from build123d import *

# Parameters (mm, degrees)
ESQUISSE1_W                     = 98
ESQUISSE1_H                     = 110
ESQUISSE1_W_2                   = 78
ESQUISSE1_H_2                   = 90
BOSS_EXTRU_1_DEPTH              = 5
ESQUISSE2_R                     = 5
ESQUISSE2_R_2                   = 2.5
BOSS_EXTRU_2_DEPTH              = 10
ESQUISSE3_R                     = 2.5
ENL_V_MAT_EXTRU_1_DEPTH         = 10
R_P_TITION_LIN_AIRE3_COUNT      = 2
R_P_TITION_LIN_AIRE3_PITCH      = 88
R_P_TITION_LIN_AIRE3_COUNT_DIR2 = 2
R_P_TITION_LIN_AIRE3_PITCH_DIR2 = 90
CONG_1_R                        = 5


with BuildPart() as part:
    # Esquisse1 → Boss.-Extru.1 (new body)
    with BuildSketch(Plane.XY):
        with Locations((54.666666667, 49.166666667)):
            Rectangle(ESQUISSE1_W, ESQUISSE1_H)
        with Locations((54.666666667, 49.166666667)):
            Rectangle(ESQUISSE1_W_2, ESQUISSE1_H_2, mode=Mode.SUBTRACT)
    extrude(amount=BOSS_EXTRU_1_DEPTH)

    # Esquisse2 → Boss.-Extru.2 (add)
    with BuildSketch(Plane(origin=(103.666666667, 0, 0), x_dir=(0, 0, -1), z_dir=(1, 0, 0))):
        with Locations((-7.1, 94.166666667)):
            Circle(ESQUISSE2_R)
        with Locations((-7.1, 94.166666667)):
            Circle(ESQUISSE2_R_2, mode=Mode.SUBTRACT)
    boss_extru_2 = extrude(amount=-BOSS_EXTRU_2_DEPTH)

    # Esquisse3 → Enlèv. mat.-Extru.1 (cut)
    with BuildSketch(Plane(origin=(103.666666667, 0, 0), x_dir=(0, 0, -1), z_dir=(1, 0, 0))):
        with Locations((-7.1, 94.166666667)):
            Circle(ESQUISSE3_R)
    enl_v_mat_extru_1 = extrude(amount=-ENL_V_MAT_EXTRU_1_DEPTH, mode=Mode.SUBTRACT)

    # Répétition linéaire3: Boss.-Extru.2, Enl_v. mat.-Extru.1 2 × 2
    with Locations(*[(-i * R_P_TITION_LIN_AIRE3_PITCH, -j * R_P_TITION_LIN_AIRE3_PITCH_DIR2, 0) for i in range(R_P_TITION_LIN_AIRE3_COUNT) for j in range(R_P_TITION_LIN_AIRE3_COUNT_DIR2) if (i, j) != (0, 0)]):
        add(boss_extru_2)
        add(enl_v_mat_extru_1, mode=Mode.SUBTRACT)

    # Congé1
    cong_1_edges = [part.edges().sort_by_distance(p)[0] for p in [
        (10.666666667, -0.370953855, 5),
        (10.666666667, 8.704287188, 5),
        (98.666666667, 89.629046145, 5),
        (98.666666667, 98.704287188, 5),
        (98.666666667, -0.370953855, 5),
        (98.666666667, 8.704287188, 5),
        (10.666666667, 89.629046145, 5),
        (10.666666667, 98.704287188, 5),
    ]]
    fillet(cong_1_edges, radius=CONG_1_R)


solid = part.part
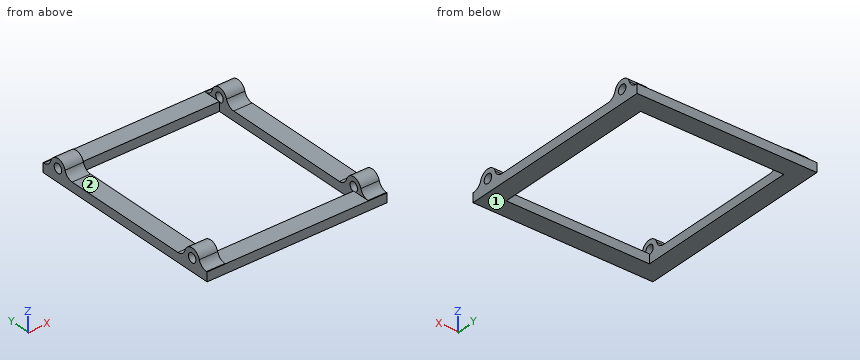
Part model, mm, in its own coordinate system. Face numbers are marked on the shaded views. Round coordinates to 2 decimals unless told otherwise and drop trailing zeros. Loops run counter-clockwise (first coordinate to the right, second up) from the corner with the lowest first, then second, coordinate; pieces in that order, holes last. Notation, with made-up numbers: (41.5, 89.5) - (85.5, 89.5) arc R23 ccw to (85.5, 113.5) - close; hole circle Ø3 at (-36.5, 59). An arc over 180 degrees is marked (long way). Answer as a JSON object with one key per item and string values.
Item 1: Band-saw the part on A-A on x = 57.5. List the corners of the cut face in (y, z).
Output:
{"outline": "(-5.83, 0) - (4.17, 0) - (4.17, 5) - (-5.83, 5) - close; (94.17, 0) - (104.17, 0) - (104.17, 5) - (94.17, 5) - close"}
Item 2: Band-saw the part on B-B on y = 49. List the corners of the cut face in (x, z), plus the area to 3 significant figures.
Output:
{"outline": "(5.67, 0) - (15.67, 0) - (15.67, 5) - (5.67, 5) - close; (93.67, 0) - (103.67, 0) - (103.67, 5) - (93.67, 5) - close", "area": "100 mm2"}
Item 3: Wall check: L1, parallel to Y at x = 88, z = 1.5; L2, parallel to X at y = 62, z = 4.5; L3, parallel to Y at x = 101, z = 7.1. Give the ranges that are in metal, low to high.
Output:
{"L1": "-5.83 to 4.17, 94.17 to 104.17", "L2": "5.67 to 15.67, 93.67 to 103.67", "L3": "-1.33 to 1.67, 6.67 to 9.66, 88.67 to 91.67, 96.67 to 99.66"}
Item 4: Band-saw the part on C-C on z = 7.1. State how many separate pieces and enclosed holes the cut face has, plus the area to 3 significant figures.
Output:
{"separate pieces": "8", "enclosed holes": "0", "area": "240 mm2"}
Item 5: Pin check, flat tips, straight feed: pin 1 (6 mm diameter, centred on y = 47, z = 6, fed in from -X); pin 2 (5 mm diameter, centred on x = 59, y = 101, fed in from +Z); pin 3 (5 mm diameter, centred on x = 93, z = 10, fed in from -Y); pin 4 (4.5 mm diameter, centred on y = 4.17, z = 7.1, fed in from +X). Stop position of each tip, or through.
Output:
{"pin 1": "x = 5.67", "pin 2": "z = 5", "pin 3": "y = -1.02", "pin 4": "x = 93.67"}
Item 6: Pull direction Y, two halves, no side cores. Call the marked faces 1 and 2: pulls with the +Y half, pulls with the -Y half, needs draft (parallel to the pull), parting line crosses it, or undercut.
Output:
{"face 1": "needs draft", "face 2": "undercut"}
